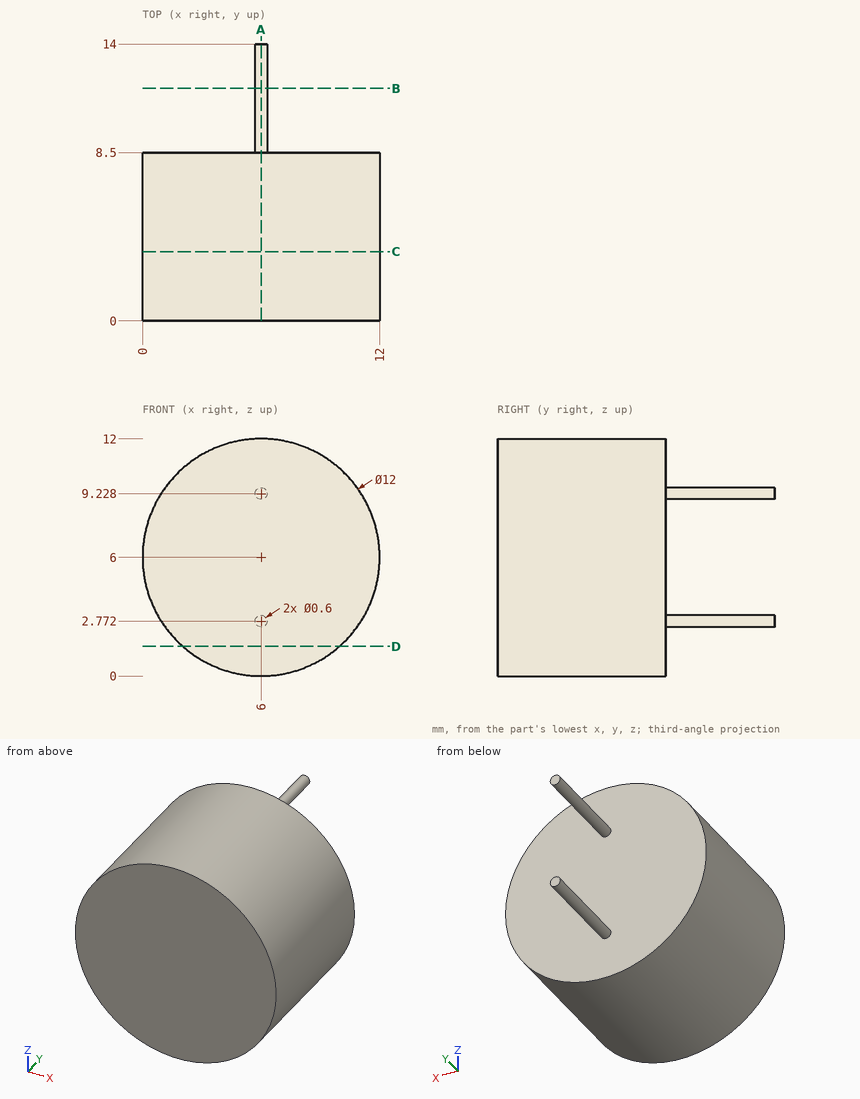
The figure shows three views and two pictorial views of one solid part (mm, origin at its lowest corner). Answer the questions. Coordinates: 2 decimals unless noted, no trailing zeros. Order: outer loops, then holes, each group sorted by start corner. A loop starts at its lowest first (then second) coordinate and runs counter-clockwise, first axis right, second up.
Q1. A cutting plane is placed at C-C, the plane y = 3.5. Write down the section's boundary in (x, z).
Q2. Given P1, Ø4, axis at y = 10, z = 8.5, coming from the -X side; P2, Ø1, axis at x = 7, z = 7.5, coming from the +Y side; P3, Ø6, axis at x = 8, z = 3.5, coming from the +Y side; P4, Ø3, axis at y = 3, z = 2, coming from the +X side, each flat-ended and moving along its own axis, determine where each tip first touches the part or whether it passes through.
Q3. Consider line 1 (Y direction, x = 1.5, z = 8.5); line 2 (Z direction, x = 3, y = 1); line 3 (X direction, y = 1, z = 10.25) (1 decimal). Determine where each line is inside the solid, lowest interval first.
Q4. A cutting plane is placed at B-B, the plane y = 11.75. Write down the section's boundary in (x, z).
Q5. A cutting plane is placed at D-D, the plane z = 1.5. Write down the section's boundary in (x, y), and give its area (3 significant figures).
Q6. A cutting plane is placed at A-A, the plane x = 6. Write down the section's boundary in (y, z), and give its area (3 significant figures).
Answers follow:
1. outline: circle Ø12 at (6, 6)
2. P1: stops at x = 0.12
2. P2: stops at y = 8.5
2. P3: stops at y = 14
2. P4: stops at x = 11.45
3. line 1: y = 0 to 8.5
3. line 2: z = 0.8 to 11.2
3. line 3: x = 1.8 to 10.2
4. outline: circle Ø0.6 at (6, 2.77); circle Ø0.6 at (6, 9.23)
5. outline: (2.03, 0) - (9.97, 0) - (9.97, 8.5) - (2.03, 8.5) - close
5. area: 67.5 mm2
6. outline: (0, 0) - (8.5, 0) - (8.5, 2.47) - (14, 2.47) - (14, 3.07) - (8.5, 3.07) - (8.5, 8.93) - (14, 8.93) - (14, 9.53) - (8.5, 9.53) - (8.5, 12) - (0, 12) - close
6. area: 109 mm2
